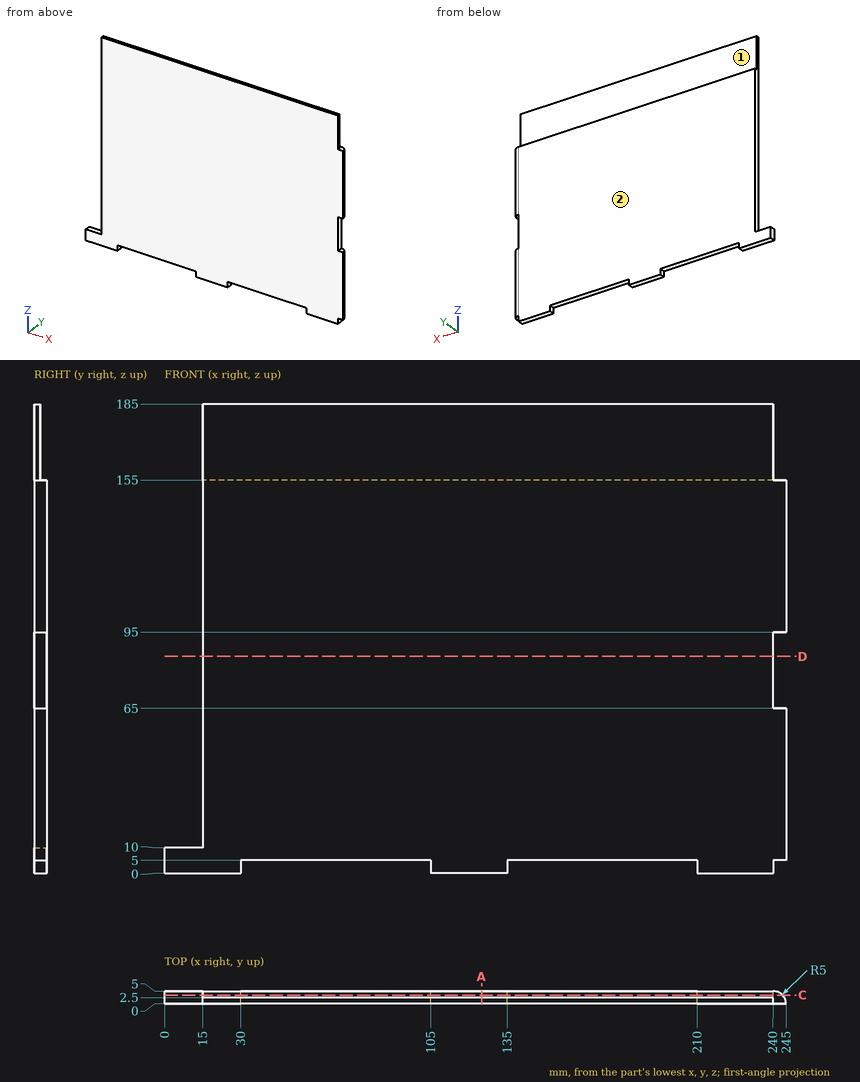
Part print with two shaded views. Sizes in mm from the minimum x, y, z corner. A direction names the side the tool comes from. Give positions to 0.01 mm unless a question says otherwise; leave off trailing zeros. Order: outer loops, then holes, each group sorted by start corner. A loop starts at its lowest first (then second) coordinate and runs counter-clockwise, first axis right, second up.
1) Saw through at D-D, the plane z = 85.5. Write the cut outline in (x, y), then the cut area to 4 significant figures.
2) Pin check, flat tips, straight feed: pin 1 (1.5 mm diameter, centred on x = 199.5, z = 165, fed in from +Y); pin 2 (1.5 mm diameter, centred on y = 2, z = 1.5, fed in from +X); pin 3 (1.5 mm diameter, centred on y = 3.5, z = 119, fed in from +X). Stop position of each tip, or through.
3) Saw through at C-C, the plane y = 3.45. Write the cut outline in (x, z).
4) Wall check: probe 1 along Z at (x, y) = (235, 3.05); probe 2 along Z at (x, y) = (38.5, 3.8); probe 3 along Y at (x, z) = (196, 172.5). Give the ranges that are in metal, low to high.
5) 3-axis set-ups, long thin cutter, end or side, ignore diameter. For the marked faces 1 and 2: which of +Z, -Z, +X, -X, +Y, -Y reach the whole face in a straight line?
6) Saw through at A-A, the plane x = 125. Write the cut outline in (y, z).
Computed:
1. outline: (15, 0) - (240, 0) - (240, 5) - (15, 5) - close
1. area: 1,125 mm2
2. pin 1: stops at y = 2.5
2. pin 2: stops at x = 240
2. pin 3: stops at x = 244.18
3. outline: (0, 0) - (30, 0) - (30, 5) - (105, 5) - (105, 0) - (135, 0) - (135, 5) - (210, 5) - (210, 0) - (240, 0) - (240, 5) - (243.62, 5) - (243.62, 65) - (240, 65) - (240, 95) - (243.62, 95) - (243.62, 155) - (15, 155) - (15, 10) - (0, 10) - close
4. probe 1: z = 0 to 155
4. probe 2: z = 5 to 155
4. probe 3: y = 0 to 2.5
5. face 1: +Z, +X, -X, +Y
5. face 2: +Z, -Z, +X, -X, +Y
6. outline: (0, 0) - (5, 0) - (5, 155) - (2.5, 155) - (2.5, 185) - (0, 185) - close
